Model file for the job. Use its own axes, mm. Face numbers are marked on the shaded views. A direction names the side the tool comes from. Coordinates: 2 decimals unless noted, no trailing zeros. Write each loop counter-clockwise with the first axis right and the second up, starting at its lowest first coordinate (ties: lowest second). Pieces come first, ordered by that corner, then holes.
Q1. Band-saw the part on A-A, the plane z = 7. Write the cut outline in (x, y), plus the area to 3 significant figures.
Q2. Pull direction Z, two halves, no side cores. Call the marked faces 4, 5, 6 and 7: released by +Z, released by -Z, zero draft, split by the parting line, or undercut.
Q3. Which spindle directions (+Z, -Z, +X, -X, +Y, -Y) get a long thin tool onto all of the face, cutting with end or side? Do the marked faces 1, 2 and 3. Say none if no direction does.
Q4. Band-saw the part on C-C, the plane z = 12. Write the cut outline in (x, y).
Q5. Band-saw the part on B-B, the plane x = 5.5. Write the cut outline in (y, z).
Q6. Pin check, flat tips, straight feed: P1, Ø4.5, axis at y = 0, z = 0, coming from the +X side; P2, Ø0.7, axis at x = 15, z = 0, coming from the +Y side; P3, Ø1, axis at y = 0.5, z = 3.5, coming from the +X side; P4, Ø8, axis at x = 13, z = 3.5, coming from the +Y side. Stop position of each tip, or through.
Q7. Drill centre lines: probe 1 along Y at (x, z) = (0, 6.5); probe 2 along Z at (x, y) = (1.1, 0); probe 3 along Y at (x, z) = (1, 0). Where is each one in solid material? Low to high.
from build123d import *

# Parameters (mm, degrees)
CUT_EXTRUDE1_DEPTH = 1.2
SKETCH6_W          = 13.5
SKETCH6_H          = 0.85
SKETCH7_W          = 16
SKETCH7_H          = 16
CUT_EXTRUDE2_DEPTH = 6.055555556


with BuildPart() as part:
    # Sketch1 → Revolve1 (revolve)
    with BuildSketch(Plane.XY):
        with BuildLine():
            Line((0, 2.8), (2.8, 2.8))
            Line((2.8, 2.8), (4, 4))
            Line((4, 4), (12.457142857, 4))
            Line((12.457142857, 4), (13.2, 3.800952028))
            Line((13.2, 3.800952028), (13.2, 3.693772352))
            Line((13.2, 3.693772352), (13.458578644, 3.693772352))
            Line((13.458578644, 3.693772352), (13.6, 3.552350995))
            Line((13.6, 3.552350995), (13.6, 2.5))
            Line((13.6, 2.5), (14.13, 2.5))
            ThreePointArc((14.13, 2.5), (14.391629509, 2.608370491), (14.5, 2.87))
            Line((14.5, 2.87), (14.5, 5.9))
            Line((14.5, 5.9), (14.897402943, 5.9))
            ThreePointArc((14.897402943, 5.9), (15.025960465, 5.853208889), (15.094364494, 5.734729636))
            Line((15.094364494, 5.734729636), (15.7, 2.3))
            Line((15.7, 2.3), (15.7, 0))
            Line((15.7, 0), (-2.8, 0))
            ThreePointArc((-2.8, 0), (-1.979898987, 1.979898987), (0, 2.8))
        make_face()
    revolve(axis=Axis((15.7, 0, 0), (-1, 0, 0)))

    # Sketch2 → Revolve2 (revolve)
    with BuildSketch(Plane(origin=(0, 0, 0), x_dir=(0, 0, -1), z_dir=(1, 0, 0))):
        Polygon((-10.5, 0), (-10.5, 3.8), (-10.1, 3.8), (-10, 3.7), (-9.9, 3.8), (-9.5, 3.8), (-9.5, 4), (-9.130495828, 4.64), (-4.869504172, 4.64), (-4.5, 4), (-4.5, 3), (-2.7, 3), (-2.5, 2.8), (0, 2.8), (0, 0), align=None)
    revolve(axis=Axis((0, 0, 0), (0, 0, 1)))

    # Sketch3 → Revolve3 (revolve)
    with BuildSketch(Plane(origin=(0, 0, 0), x_dir=(0, 0, -1), z_dir=(1, 0, 0))):
        Polygon((-13.5, 0), (-13.5, 2.0095), (-13.0095, 2.5), (-10.5, 2.5), (-10.5, 0), align=None)
    revolve(axis=Axis((0, 0, 10.5), (0, 0, 1)))

    # Sketch4 → Cut-Extrude1 (cut)
    with BuildSketch(Plane(origin=(15.7, 0, 0), x_dir=(0, 0, -1), z_dir=(1, 0, 0))):
        Polygon((-9.8, -5.658032638), (0, -11.316065276), (9.8, -5.658032638), (9.8, 5.658032638), (0, 11.316065276), (-9.8, 5.658032638), align=None)
        with BuildLine():
            Line((-1, -3.9), (1, -3.9))
            ThreePointArc((1, -3.9), (4.9, 0), (1, 3.9))
            Line((1, 3.9), (-1, 3.9))
            ThreePointArc((-1, 3.9), (-4.9, 0), (-1, -3.9))
        make_face(mode=Mode.SUBTRACT)
    extrude(amount=-CUT_EXTRUDE1_DEPTH, mode=Mode.SUBTRACT)

    # Sketch6 → Cut-Revolve1 (revolve, cut)
    with BuildSketch(Plane(origin=(0, 0, 0), x_dir=(0, 0, -1), z_dir=(1, 0, 0))):
        with Locations((-6.75, 0.425)):
            Rectangle(SKETCH6_W, SKETCH6_H)
    revolve(axis=Axis((0, 0, 0), (0, 0, 1)), mode=Mode.SUBTRACT)

    # Sketch5 → Cut-Revolve2 (revolve, cut)
    with BuildSketch(Plane(origin=(0, 0, 0), x_dir=(1, 0, 0), z_dir=(0, 1, 0))):
        with BuildLine():
            Line((0, 0.85), (4.1, 0.85))
            Line((4.1, 0.85), (4.1, 2))
            Line((4.1, 2), (15.4, 2))
            ThreePointArc((15.4, 2), (15.612132034, 2.087867966), (15.7, 2.3))
            Line((15.7, 2.3), (15.7, 0))
            Line((15.7, 0), (-0.85, 0))
            ThreePointArc((-0.85, 0), (-0.601040764, 0.601040764), (0, 0.85))
        make_face()
    revolve(axis=Axis((15.7, 0, 0), (-1, 0, 0)), mode=Mode.SUBTRACT)

    # Sketch7 → Cut-Extrude2 (cut)
    with BuildSketch(Plane.XY.offset(10.5)):
        Rectangle(SKETCH7_W, SKETCH7_H)
        Polygon((-4.618802154, 0), (-2.309401077, -4), (2.309401077, -4), (4.618802154, 0), (2.309401077, 4), (-2.309401077, 4), align=None, mode=Mode.SUBTRACT)
    extrude(amount=-CUT_EXTRUDE2_DEPTH, mode=Mode.SUBTRACT)


solid = part.part
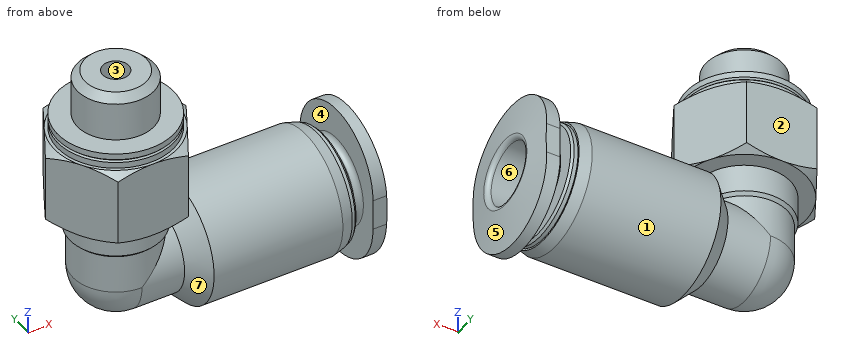
Answer sheet:
1. outline: (-4.62, 0) - (-2.31, -4) - (2.31, -4) - (4.62, 0) - (2.31, 4) - (-2.31, 4) - close; hole circle Ø1.7 at (0, 0)
1. area: 53.2 mm2
2. face 4: zero draft
2. face 5: split by the parting line
2. face 6: undercut
2. face 7: undercut
3. face 1: none
3. face 2: +Z, -Z, +X, -X, +Y
3. face 3: +Z
4. outline: circle Ø5 at (0, 0); hole circle Ø1.7 at (0, 0)
5. outline: circle Ø8 at (0, 0); hole circle Ø4 at (0, 0)
6. P1: stops at x = 15.7
6. P2: stops at y = 3.9
6. P3: stops at x = 15.57
6. P4: stops at y = 4
7. probe 1: y = -4 to -0.85, 0.85 to 4
7. probe 2: z = -2.8 to -0.85, 0.85 to 13.5
7. probe 3: y = -2.8 to -0.85, 0.85 to 2.8
